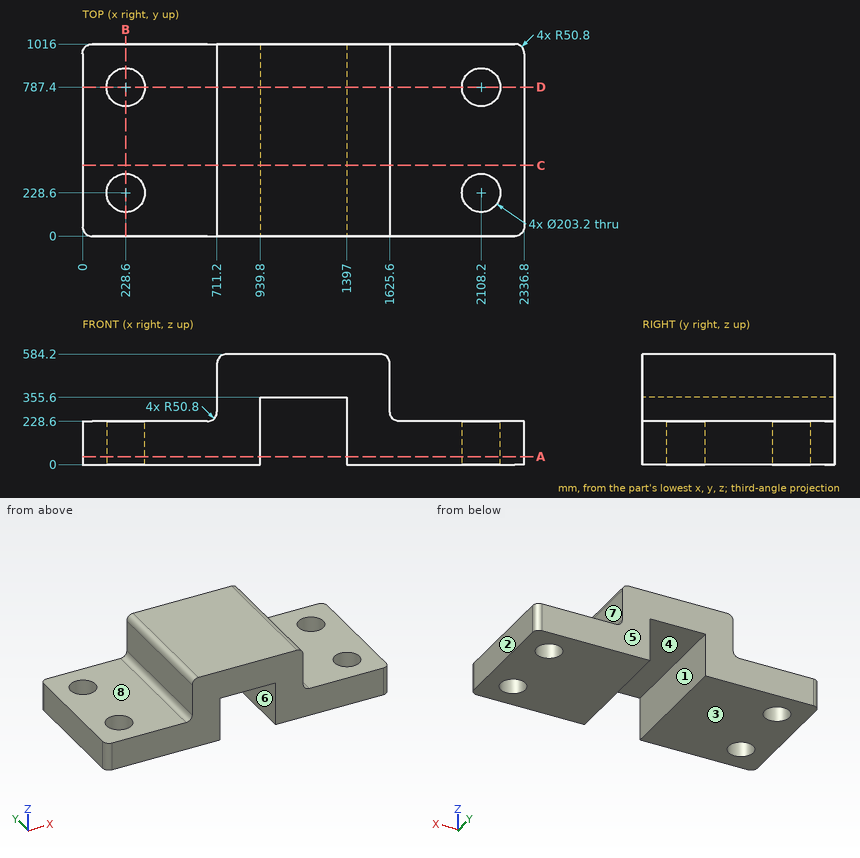
Source: three-view drawing plus pictorial views. Frame: mm from the lowest corner of the part. A direction names the side the tool comes from. Give positions to 0.01 mm unless a question says otherwise; leave off trailing zeros. Order: outer loops, then holes, each group sorted by start corner. A loop starts at its lowest first (then second) coordinate and runs counter-clockwise, first axis right, second up. Notation, with made-up numbers: M 46,-1.5 L 56,-1.5 A7 cw 56,8.5 Z; hole C 18,6.5 d4. An arc over 180 degrees is marked long. Return JSON: item names as keys, results as strings.
Item 1: Cut plane D-D (y = 787.4). Return loops of the section in (x, z), then the cut area to 3 significant figures.
Solutions:
{"outline": "M 0,0 L 127,0 L 127,228.6 L 0,228.6 Z; M 330.2,0 L 939.8,0 L 939.8,355.6 L 1397,355.6 L 1397,0 L 2006.6,0 L 2006.6,228.6 L 1676.4,228.6 A50.8 cw 1625.6,279.4 L 1625.6,533.4 A50.8 ccw 1574.8,584.2 L 762,584.2 A50.8 ccw 711.2,533.4 L 711.2,279.4 A50.8 cw 660.4,228.6 L 330.2,228.6 Z; M 2209.8,0 L 2336.8,0 L 2336.8,228.6 L 2209.8,228.6 Z", "area": "604,000 mm^2"}
Item 2: First-contact query: P1, Ø10, axis at x = 1085, y = 701.5, coming from the -Z side; P2, Ø6, axis at y = 711.5, z = 249, coming from the -X side; P3, Ø8, axis at y = 531, z = 503.5, coming from the -X side. Flat tips, straight axial feed; report the tip coordinate or a pass-through.
Solutions:
{"P1": "z = 355.6", "P2": "x = 698.68", "P3": "x = 711.2"}
Item 3: Ray query, probe 1 along Y at (x, z) = (2108, 171); probe 2 along X at (y, z) = (787.4, 158.5); probe 3 along X at (y, z) = (707, 206). Return the intervals inside material, ascending.
Solutions:
{"probe 1": "0 to 127, 330.2 to 685.8, 889 to 1016", "probe 2": "0 to 127, 330.2 to 939.8, 1397 to 2006.6, 2209.8 to 2336.8", "probe 3": "0 to 166.48, 290.72 to 939.8, 1397 to 2046.08, 2170.32 to 2336.8"}
Item 4: Pull-direction query (X, two-part tool) for the marked faces 1, 2, 3 and 4; classes: +X half, -X half, draft (parallel to the pull), parting line (faces both ways), or undercut.
Solutions:
{"face 1": "undercut", "face 2": "+X half", "face 3": "draft", "face 4": "undercut"}
Item 5: Cut plane C-C (y = 373.5). Return loops of the section in (x, z), then the cut area to 3 significant figures.
Solutions:
{"outline": "M 0,0 L 939.8,0 L 939.8,355.6 L 1397,355.6 L 1397,0 L 2336.8,0 L 2336.8,228.6 L 1676.4,228.6 A50.8 cw 1625.6,279.4 L 1625.6,533.4 A50.8 ccw 1574.8,584.2 L 762,584.2 A50.8 ccw 711.2,533.4 L 711.2,279.4 A50.8 cw 660.4,228.6 L 0,228.6 Z", "area": "697,000 mm^2"}
Item 6: Cut plane B-B (x = 228.6). Return loops of the section in (y, z), then the cut area to 3 significant figures.
Solutions:
{"outline": "M 0,0 L 127,0 L 127,228.6 L 0,228.6 Z; M 330.2,0 L 685.8,0 L 685.8,228.6 L 330.2,228.6 Z; M 889,0 L 1016,0 L 1016,228.6 L 889,228.6 Z", "area": "139,000 mm^2"}
Item 7: Cut plane A-A (z = 42). Return loops of the section in (x, y).
Solutions:
{"outline": "M 0,50.8 A50.8 ccw 50.8,0 L 939.8,0 L 939.8,1016 L 50.8,1016 A50.8 ccw 0,965.2 Z; M 1397,0 L 2286,0 A50.8 ccw 2336.8,50.8 L 2336.8,965.2 A50.8 ccw 2286,1016 L 1397,1016 Z; hole C 228.6,228.6 d203.2; hole C 228.6,787.4 d203.2; hole C 2108.2,228.6 d203.2; hole C 2108.2,787.4 d203.2"}
Item 8: Access query for the marked faces 5, 6, 7 and 8. Directions: +Z, -Z, +X, -X, +Y, -Y. A direction counts if a zero-diameter tool reaches every point of the face in a straight line with its end or side. Return the directions, or none.
Solutions:
{"face 5": "+Z, -Z, +X, -X, +Y", "face 6": "-Z, +Y, -Y", "face 7": "+Z, +X, +Y, -Y", "face 8": "+Z, -X, +Y, -Y"}
